Source: CAD feature listing. Evaluate the final solid. Frame: model axes, mm. Face numbers are marked on the shaded views. Round coordinates to 2 decimals unless told otherwise and drop trailing zeros. Order: outer loops, then holes, each group sorted by start corner. A loop starts at its lowest first (then second) coordinate and runs counter-clockwise, first axis right, second up.
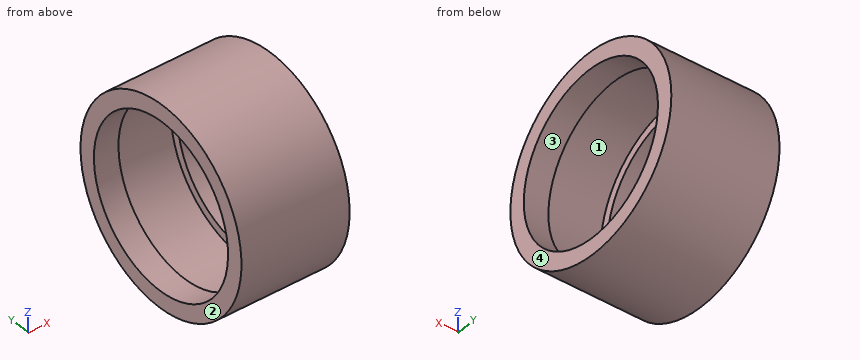
Autodesk Inventor part; units mm, degrees
ref_plane "YZ Plane" through (0, 0, 0) normal (1, 0, 0) x (0, 1, 0)
ref_plane "XZ Plane" through (0, 0, 0) normal (0, 1, 0) x (-1, 0, 0)
ref_plane "XY Plane" through (0, 0, 0) normal (0, 0, 1) x (1, 0, 0)
sketch "Sketch1" plane through (0, 0, 0) normal (1, 0, 0) x (0, 1, 0)
  circle A0 centre (0, 0) radius 12
  circle A1 centre (0, 0) radius 11
  dimension "d0" = 24
  dimension "d1" = 22
extrude "Extrusion1" add sketch "Sketch1" along normal mid plane 13.2
sketch "Sketch4" plane through (-6.6, 0, 0) normal (-1, 0, 0) x (0, 0, 1)
  circle A0 centre (0, 0) radius 10
  circle A1 centre (0, 0) radius 11
  dimension "d9" = 20
  dimension "d10" = 22
extrude "Extrusion3" add sketch "Sketch4" against normal blind 3
sketch "Sketch5" plane through (6.6, 0, 0) normal (1, 0, 0) x (0, 0, -1)
  circle A0 centre (0, 0) radius 10
  circle A1 centre (0, 0) radius 11
  dimension "d13" = 20
  dimension "d14" = 22
extrude "Extrusion4" add sketch "Sketch5" against normal blind 3
equation "\"d0\" = BearingDiameter"
equation "\"d2\" = BearingSiliconeWidth"
properties part number "Bearing_Silicone" material "UHMW, White"
1. Line query: line 1 along Z through (x, y) = (-0.5, 0); line 2 along Y through (x, z) = (-2.25, 7.5); line 3 along Z through (x, y) = (-1.25, -7). Output: solid intervals per line, ascending.
2. Section A-A on z = 0. Return loops of the section in (x, y), plus the area to 3 significant figures.
3. Section D-D on x = -5.25. Return loops of the section in (y, z), plus the area to 3 significant figures.
4. Pull-direction query (X, two-part tool) for the marked faces 1, 2, 3 and 4; classes: released by +X, released by -X, zero draft, split by the parting line, or undercut.
5. Section C-C on x = 0.25. Return loops of the section in (y, z).
6. First-contact query: pin 1 (6 mm diameter, centred on x = 3.5, z = -8, fed in from +Y); pin 2 (2 mm diameter, centred on x = -4, z = 9.5, fed in from -Y); pin 3 (2 mm diameter, centred on x = 1, z = -7.5, fed in from +Y); pin 4 (10 mm diameter, centred on y = -1, z = 0.5, fed in from +X) (1 decimal). Flat tips, straight axial feed; report the tip coordinate or a pass-through.
Result:
1. line 1: z = -12 to -11, 11 to 12
1. line 2: y = -9.37 to -8.05, 8.05 to 9.37
1. line 3: z = -9.75 to -8.49, 8.49 to 9.75
2. outline: (-6.6, -12) - (6.6, -12) - (6.6, -10) - (3.6, -10) - (3.6, -11) - (-3.6, -11) - (-3.6, -10) - (-6.6, -10) - close; (-6.6, 10) - (-3.6, 10) - (-3.6, 11) - (3.6, 11) - (3.6, 10) - (6.6, 10) - (6.6, 12) - (-6.6, 12) - close
2. area: 38.4 mm2
3. outline: circle Ø24 at (0, 0); hole circle Ø20 at (0, 0)
3. area: 138 mm2
4. face 1: undercut
4. face 2: released by -X
4. face 3: zero draft
4. face 4: released by +X
5. outline: circle Ø24 at (0, 0); hole circle Ø22 at (0, 0)
6. pin 1: stops at y = 10.91
6. pin 2: stops at y = -8.47
6. pin 3: stops at y = 10.09
6. pin 4: passes through
